from build123d import *

# Parameters (mm, degrees)
F1_DEPTH     = 25.4
F2_T1_DEPTH  = 25.4
F2_T3_DEPTH  = 196.85
F2_T5_DEPTH  = 88.9
F2_T10_DEPTH = 241.3
F2_T15_DEPTH = 241.3
F2_T18_ANGLE = 233.2969892374
F2_T20_ANGLE = 233.2969892374
F3_C1_SIZE   = 12.7
F3_C2_SIZE   = 12.7
F3_C3_SIZE   = 12.6999
F3_C4_SIZE   = 12.6999


# Not quite as in the source:
# - a fillet or chamfer that OpenCascade refuses, or shapes differently, is made with other operations: its cross-section is extruded or revolved along the edge and cut away or added
# - a fillet or chamfer is up to 0.001 mm smaller than in the source, because OpenCascade refuses the exact size


with BuildPart() as f1:
    # F0 (on Front) → F1 (new body)
    with BuildSketch(Plane.XZ):
        Polygon((-25.4, -107.4178270914), (0, -107.4178270914), (25.4, -107.4178270914), (25.4, 70.3821729086), (-25.4, 70.3821729086), align=None)
        with BuildLine():
            ThreePointArc((-31.8772674395, 83.0821729086), (-28.6865783939, 76.7077201152), (-25.4, 70.3821729086))
            Line((-25.4, 70.3821729086), (25.4, 70.3821729086))
            Line((25.4, 70.3821729086), (46.7168006713, 61.0254222331))
            ThreePointArc((46.7168006713, 61.0254222331), (8.0726901659, 114.8632107301), (-21.8660467054, 173.9863600165))
            ThreePointArc((-21.8660467054, 173.9863600165), (-51.7756284743, 387.4903570682), (25.4, 588.7922751123))
            ThreePointArc((25.4, 588.7922751123), (-77.2246025315, 344.3169540256), (-31.8772674395, 83.0821729086))
        make_face()
        with BuildLine():
            Line((-38.1, 70.3821729086), (-25.4, 70.3821729086))
            ThreePointArc((-25.4, 70.3821729086), (-28.6865783939, 76.7077201152), (-31.8772674395, 83.0821729086))
            Line((-31.8772674395, 83.0821729086), (-38.1, 83.0821729086))
            Line((-38.1, 83.0821729086), (-38.1, 70.3821729086))
        make_face()
        with BuildLine():
            ThreePointArc((-21.8660467054, 173.9863600165), (8.0726901659, 114.8632107301), (46.7168006713, 61.0254222331))
            Line((46.7168006713, 61.0254222331), (121.4661896229, 28.2150860876))
            ThreePointArc((121.4661896229, 28.2150860876), (42.125694257, 93.5547531424), (-21.8660467054, 173.9863600165))
        make_face()
    extrude(amount=F1_DEPTH)

    # F2: fillet of radius 12.7 on 6 edges, made by hand

    # F2_s2 → F2_t1 (join)
    with BuildSketch(Plane.XZ):
        with BuildLine():
            ThreePointArc((-25.4, 57.6821729086), (-29.1197438789, 66.6624290297), (-38.1, 70.3821729086))
            Line((-38.1, 70.3821729086), (-25.4, 70.3821729086))
            Line((-25.4, 70.3821729086), (-25.4, 57.6821729086))
        make_face()
    extrude(amount=F2_T1_DEPTH)

    # F2_s4 → F2_t3 (cut)
    with BuildSketch(Plane.XY.offset(-139.1678270914)):
        with BuildLine():
            ThreePointArc((-25.4, -12.7), (-21.6802561211, -3.7197438789), (-12.7, 0))
            Line((-12.7, 0), (-25.4, 0))
            Line((-25.4, 0), (-25.4, -12.7))
        make_face()
        with BuildLine():
            ThreePointArc((-25.4, -12.7), (-21.6802561211, -21.6802561211), (-12.7, -25.4))
            Line((-12.7, -25.4), (-25.4, -25.4))
            Line((-25.4, -25.4), (-25.4, -12.7))
        make_face()
    extrude(amount=F2_T3_DEPTH, mode=Mode.SUBTRACT)

    # F2_s6 → F2_t5 (cut)
    with BuildSketch(Plane.XZ.offset(-31.75)):
        with BuildLine():
            ThreePointArc((-25.4, -94.7178270914), (-21.6802561211, -103.6980832124), (-12.7, -107.4178270914))
            Line((-12.7, -107.4178270914), (-25.4, -107.4178270914))
            Line((-25.4, -107.4178270914), (-25.4, -94.7178270914))
        make_face()
    extrude(amount=F2_T5_DEPTH, mode=Mode.SUBTRACT)


with BuildPart() as f2_tool8:
    # F2_s9 → F2_t10 (new body)
    with BuildSketch(Plane.XY.offset(-139.1678270914)):
        with BuildLine():
            ThreePointArc((12.7, 0), (21.6802561211, -3.7197438789), (25.4, -12.7))
            Line((25.4, -12.7), (25.4, 0))
            Line((25.4, 0), (12.7, 0))
        make_face()
    extrude(amount=F2_T10_DEPTH)

    split(bisect_by=Plane(origin=(30.005981648, 0, 68.3604332226), x_dir=(0, 1, 0), z_dir=(-0.4019236244, 0, -0.9156731951)), keep=Keep.TOP)


with BuildPart() as f1_1:
    add(f1.part)

    # F2_t7: cut F2_tool8
    add(f2_tool8.part, mode=Mode.SUBTRACT)


with BuildPart() as f2_tool13:
    # F2_s14 → F2_t15 (new body)
    with BuildSketch(Plane.XY.offset(-139.1678270914)):
        with BuildLine():
            ThreePointArc((12.7, -25.4), (21.6802561211, -21.6802561211), (25.4, -12.7))
            Line((25.4, -12.7), (25.4, -25.4))
            Line((25.4, -25.4), (12.7, -25.4))
        make_face()
    extrude(amount=F2_T15_DEPTH)

    split(bisect_by=Plane(origin=(30.005981648, 0, 68.3604332226), x_dir=(0, 1, 0), z_dir=(-0.4019236244, 0, -0.9156731951)), keep=Keep.TOP)


with BuildPart() as f1_2:
    add(f1_1.part)

    # F2_t12: cut F2_tool13
    add(f2_tool13.part, mode=Mode.SUBTRACT)

    # F2_s17 → F2_t18 (revolve, cut)
    with BuildSketch(Plane.XY.offset(57.6821729086)):
        with BuildLine():
            ThreePointArc((-12.7, -25.4), (-21.6802561211, -21.6802561211), (-25.4, -12.7))
            Line((-25.4, -12.7), (-25.4, -25.4))
            Line((-25.4, -25.4), (-12.7, -25.4))
        make_face()
    revolve(axis=Axis((-38.1, -25.4, 57.6821729086), (0, -1, 0)), revolution_arc=F2_T18_ANGLE, mode=Mode.SUBTRACT)

    # F2_s19 → F2_t20 (revolve, cut)
    with BuildSketch(Plane.XY.offset(57.6821729086)):
        with BuildLine():
            ThreePointArc((-12.7, 0), (-21.6802561211, -3.7197438789), (-25.4, -12.7))
            Line((-25.4, -12.7), (-25.4, 0))
            Line((-25.4, 0), (-12.7, 0))
        make_face()
    revolve(axis=Axis((-38.1, 0, 57.6821729086), (0, -1, 0)), revolution_arc=F2_T20_ANGLE, mode=Mode.SUBTRACT)

    # F3: chamfer of 12.7 on 4 edges, made by hand

    # F3_c1
    f3_c1_edges = [f1_2.edges().sort_by_distance(p)[0] for p in [
        (-51.7756284743, 0, 387.4903570682),
    ]]
    chamfer(f3_c1_edges, length=F3_C1_SIZE)

    # F3_c2
    f3_c2_edges = [f1_2.edges().sort_by_distance(p)[0] for p in [
        (42.125694257, 0, 93.5547531424),
    ]]
    chamfer(f3_c2_edges, length=F3_C2_SIZE)

    # F3_c3 (size 12.7 in the source; OpenCascade refuses exactly that, so slightly less here)
    f3_c3_edges = [f1_2.edges().sort_by_distance(p)[0] for p in [
        (-51.7756284743, -25.4, 387.4903570682),
    ]]
    chamfer(f3_c3_edges, length=F3_C3_SIZE)

    # F3_c4 (size 12.7 in the source; OpenCascade refuses exactly that, so slightly less here)
    f3_c4_edges = [f1_2.edges().sort_by_distance(p)[0] for p in [
        (42.125694257, -25.4, 93.5547531424),
    ]]
    chamfer(f3_c4_edges, length=F3_C4_SIZE)


solid = f1_2.part
For this review, take the finished solid that the model builds, in its own axes (mm). A direction names the side the tool comes from. Round coordinates to 2 decimals unless told otherwise and drop trailing zeros. Order: outer loops, then holes, each group sorted by start corner. A loop starts at its lowest first (then second) coordinate and runs counter-clockwise, first axis right, second up. Notation, with made-up numbers: (73, 70) -> (99, 70) arc R22 ccw to (99, 82) -> close; hole circle Ø6 at (17, 15). An arc over 180 degrees is marked (long way). Write item = value, one per line. Start each with the question number.
1) Tool access review of faces 4 (the face through (-38.1, -13, 78)), 5 (the face through (-55.153, -12.083, 335.447)): name each direction out of +Z, -Z, +X, -X, +Y, -Y from which nothing blocks a thin tool from reaching the whole face with its end or side.
2) To check wall thickness, follow line 1 (Z direction, x = -5, y = -15.5); line 2 (X direction, y = -15.25, z = 354); line 3 (X direction, y = -22.25, z = -8). State the ranges of each line that lie inside material, in increasing order. Write a range as from..to.
3) Take a section at B-B on y = -6.25. State the section outline as (x, z) points, plus the area to 3 significant figures.
4) Insertion check: pin 1 (5 mm diameter, centred on x = -9.5, y = -7, fed in from +Z); pin 2 (1 mm diameter, centred on x = 32.5, y = -18.5, fed in from +Z); pin 3 (1.5 mm diameter, centred on y = -18.5, z = 42.5, fed in from -X). Each pin has a flat end and moves straight along its axis. Give the tip position at first contact, or say it passes through.
5) The part is to be moulded in two halves that separate along Z. For faces 1 (the face through (-55.153, -13.317, 335.447)), 2 (the face through (-22, -25.4, 109)), 3 (the face through (-20.1, -12.52, -105.04)), say which applies: +Z half, -Z half, draft (parallel to the pull), parting line (faces both ways), or undercut.
6) Take a section at A-A on z = 22. State the section outline as (x, y) points.
Verdict:
q1.face_4 = -Z, -X, +Y, -Y
q1.face_5 = +X, +Y
q2.line_1 = -107.42..144.47, 545.31..546.85
q2.line_2 = -76.03..-56.83
q2.line_3 = -21.07..21.07
q3.outline = (-38.1, 72.14) arc R14.46 cw to (-23.64, 57.68) -> (-23.64, -101.17) arc R12.7 ccw to (-12.7, -107.42) -> (23.64, -107.42) -> (23.64, 71.15) -> (92.08, 41.12) arc R497.22 cw to (-27.61, 171) arc R437.69 cw to (-24.4, 513.87) arc R472.07 ccw to (-31.88, 83.08) -> (-38.1, 83.08) -> close
q3.area = 20,700 mm2
q4.pin_1 = 542.53
q4.pin_2 = 96.06
q4.pin_3 = -24.35
q5.face_1 = undercut
q5.face_2 = draft
q5.face_3 = -Z half
q6.outline = (-12.7, -25.4) -> (12.7, -25.4) arc R12.7 ccw to (12.7, 0) -> (-12.7, 0) arc R12.7 ccw to start
